```python
from build123d import *

# Parameters (mm, degrees)
SKETCH2_R          = 1.8288
CUT_EXTRUDE1_DEPTH = 9.7754
SKETCH3_R          = 1.8288
CUT_EXTRUDE2_DEPTH = 9.7754001
CUT_EXTRUDE3_DEPTH = 3.6576


with BuildPart() as part:
    # Sketch1 → Revolve1 (revolve)
    with BuildSketch(Plane(origin=(0, 0, 0), x_dir=(0, 0, -1), z_dir=(1, 0, 0)), mode=Mode.PRIVATE) as revolve1_sk:
        Polygon((0, 5.725), (0, 4.225), (7.802, 4.225), (7.802, 7.2754), (20.802, 7.2754), (20.802, 8.7754), (6.802, 8.7754), (6.802, 6.35), (4.262, 6.35), (4.262, 5.725), align=None)
    revolve(revolve1_sk.sketch.rotate(Axis((0, 0, 0), (0, 0, 1)), 90), axis=Axis((0, 0, 0), (0, 0, 1)))  # turned: the seam where the file's is

    # Sketch2 → Cut-Extrude1 (cut, through all)
    with BuildSketch(Plane(origin=(0, 0, 0), x_dir=(1, 0, 0), z_dir=(0, 1, 0))):
        with Locations(Location((0, 11.802, 0), (0, 0, 90))):  # turned: the seam where the file's is
            Circle(SKETCH2_R)
    extrude(amount=CUT_EXTRUDE1_DEPTH, mode=Mode.SUBTRACT)

    # Sketch3 → Cut-Extrude2 (cut, through all)
    with BuildSketch(Plane(origin=(0, 0, 0), x_dir=(0, 0, -1), z_dir=(1, 0, 0))):
        with Locations((11.802, 0)):
            Circle(SKETCH3_R)
    extrude(amount=-CUT_EXTRUDE2_DEPTH, mode=Mode.SUBTRACT)

    # Sketch4 → Cut-Extrude3 (cut)
    with BuildSketch(Plane(origin=(0, 0, -9.9732), x_dir=(-1, 0, 0), z_dir=(0, 0, -1))):
        with BuildLine():
            Line((0, 0), (0, 8.7754))
            ThreePointArc((0, 8.7754), (6.205144848, 6.205144848), (8.7754, 0))
            Line((8.7754, 0), (0, 0))
        make_face()
    extrude(amount=CUT_EXTRUDE3_DEPTH, mode=Mode.SUBTRACT)


solid = part.part
```
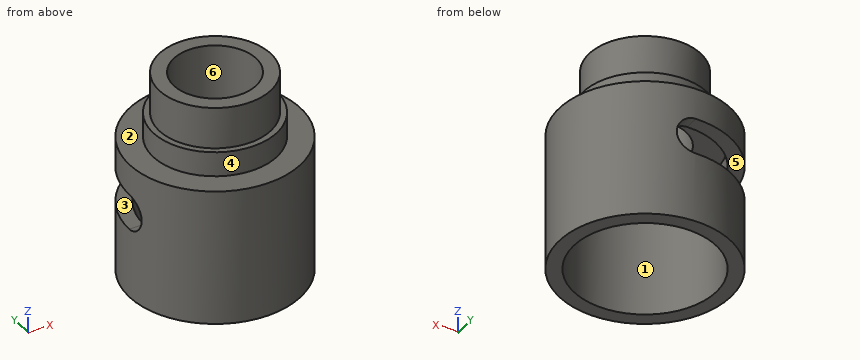
Input: part model. Units: mm. Frame: model coordinates. Face numbers are marked on the shaded views. A direction names the side the tool comes from. Coordinates: 2 decimals unless noted, no trailing zeros. Loops run counter-clockwise (first coordinate to the right, second up) from the corner with the lowest first, then second, coordinate; pieces in that order, holes last.
Q1. Set-up query: the marked faces 1, 2 and 3. Return all of +Z, -Z, +X, -X, +Y, -Y with unobstructed straight access to the full face (end or side cutting, diameter ignored); none if empty.
Results are:
face 1: -Z
face 2: +Z
face 3: -X, +Y
Q2. Section B-B, the plane z = -3. Return the cut outline in (x, y) (3 decimals), and give its area (3 significant figures).
Results are:
outline: circle Ø11.45 at (0, 0); hole circle Ø8.45 at (0, 0)
area: 46.9 mm2
Q3. Line query: line 1 along Y through (x, z) = (0, -3.75) (3 decimals); line 2 along Y through (x, z) = (0, -14); line 3 along Z through (x, y) = (5.5, -2). Output: solid intervals per line, ascending.
Results are:
line 1: y = -5.725 to -4.225, 4.225 to 5.725
line 2: y = -8.78 to -7.28, 7.28 to 8.78
line 3: z = -7.8 to -4.26
Q4. Mould query, pull axis Y, two halves, no side actions, for the marked faces 4, 5 and 6. Classes: +Y half, -Y half, draft (parallel to the pull), parting line (faces both ways), or undercut.
Results are:
face 4: parting line
face 5: draft
face 6: undercut
Q5. Section A-A, the plane z = -6.25. Return the cut outline in (x, y) (3 decimals).
Results are:
outline: circle Ø12.7 at (0, 0); hole circle Ø8.45 at (0, 0)
Q6. Contact query for flat-ended pins moving along their axis: pin 1 (2 mm diameter, centred on x = 4, z = -7, fed in from +Y); pin 2 (4 mm diameter, centred on x = 3.5, y = -0.5, fed in from -Z); pin 3 (6 mm diameter, centred on y = 6, z = -17, fed in from +X). Output: stop coordinate, or through.
Results are:
pin 1: stops at y = 8.25
pin 2: stops at z = -7.8
pin 3: stops at x = 8.25
